```python
from build123d import *

# Parameters (mm, degrees)
SKETCH_2_W          = 60
SKETCH_2_H          = 95
EXTRUDE_1_DEPTH     = 45
SKETCH_3_W          = 56
SKETCH_3_H          = 91
CUT_EXTRUDE_1_DEPTH = 40
SKETCH_5_W          = 51
SKETCH_5_H          = 70
CUT_EXTRUDE_2_DEPTH = 5
SKETCH_6_R          = 1.5
CUT_EXTRUDE_3_DEPTH = 5
SKETCH_8_R          = 2.75
CUT_EXTRUDE_4_DEPTH = 2.5
SKETCH_10_W         = 36
SKETCH_10_H         = 3
CUT_EXTRUDE_5_DEPTH = 2
SKETCH_11_W         = 60
SKETCH_11_H         = 95
EXTRUDE_2_DEPTH     = 5
SKETCH_12_W         = 56
SKETCH_12_H         = 91
CUT_EXTRUDE_6_DEPTH = 5
SKETCH_13_W         = 9
SKETCH_13_H         = 11
CUT_EXTRUDE_7_DEPTH = 5
SKETCH_14_W         = 22
SKETCH_14_H         = 19
EXTRUDE_3_DEPTH     = 31
SKETCH_15_W         = 20
SKETCH_15_H         = 17
CUT_EXTRUDE_8_DEPTH = 30
SKETCH_16_W         = 16
SKETCH_16_H         = 14
CUT_EXTRUDE_9_DEPTH = 2


with BuildPart() as part:
    # 草圖2 → 填料-伸長1 (new body)
    with BuildSketch(Plane(origin=(0, 0, 0), x_dir=(1, 0, 0), z_dir=(0, 1, 0))):
        with Locations((30, 47.5)):
            Rectangle(SKETCH_2_W, SKETCH_2_H)
    extrude(amount=EXTRUDE_1_DEPTH)

    # 草圖3 → 除料-伸長1 (cut)
    with BuildSketch(Plane(origin=(0, 45, 0), x_dir=(1, 0, 0), z_dir=(0, 1, 0))):
        with Locations((30, 47.5)):
            Rectangle(SKETCH_3_W, SKETCH_3_H)
    extrude(amount=-CUT_EXTRUDE_1_DEPTH, mode=Mode.SUBTRACT)

    # 草圖5 → 除料-伸長2 (cut)
    with BuildSketch(Plane(origin=(0, 5, 0), x_dir=(1, 0, 0), z_dir=(0, 1, 0))):
        with Locations((30, 46.5)):
            Rectangle(SKETCH_5_W, SKETCH_5_H)
    extrude(amount=-CUT_EXTRUDE_2_DEPTH, mode=Mode.SUBTRACT)

    # 草圖6 → 除料-伸長3 (cut)
    with BuildSketch(Plane(origin=(0, 5, 0), x_dir=(1, 0, 0), z_dir=(0, 1, 0))):
        with Locations(Location((8, 8.5, 0), (0, 0, 270))):  # turned: the seam where the file's is
            Circle(SKETCH_6_R)
        with Locations(Location((52, 8.5, 0), (0, 0, 270))):  # turned: the seam where the file's is
            Circle(SKETCH_6_R)
        with Locations(Location((8, 84.5, 0), (0, 0, 270))):  # turned: the seam where the file's is
            Circle(SKETCH_6_R)
        with Locations(Location((52, 84.5, 0), (0, 0, 270))):  # turned: the seam where the file's is
            Circle(SKETCH_6_R)
    extrude(amount=-CUT_EXTRUDE_3_DEPTH, mode=Mode.SUBTRACT)

    # 草圖8 → 除料-伸長4 (cut)
    with BuildSketch(Plane(origin=(0, 0, 0), x_dir=(-1, 0, 0), z_dir=(0, -1, 0))):
        with Locations(Location((-8, 84.5, 0), (0, 0, 90))):  # turned: the seam where the file's is
            Circle(SKETCH_8_R)
        with Locations(Location((-8, 8.5, 0), (0, 0, 90))):  # turned: the seam where the file's is
            Circle(SKETCH_8_R)
        with Locations(Location((-52, 8.5, 0), (0, 0, 90))):  # turned: the seam where the file's is
            Circle(SKETCH_8_R)
        with Locations(Location((-52, 84.5, 0), (0, 0, 90))):  # turned: the seam where the file's is
            Circle(SKETCH_8_R)
    extrude(amount=-CUT_EXTRUDE_4_DEPTH, mode=Mode.SUBTRACT)

    # 草圖10 → 除料-伸長5 (cut)
    with BuildSketch(Plane(origin=(0, 5, 0), x_dir=(1, 0, 0), z_dir=(0, 1, 0))):
        with Locations((30, 89.5)):
            Rectangle(SKETCH_10_W, SKETCH_10_H)
    extrude(amount=-CUT_EXTRUDE_5_DEPTH, mode=Mode.SUBTRACT)

    # 草圖11 → 填料-伸長2 (add)
    with BuildSketch(Plane.XZ.offset(-45)):
        with Locations((30, -47.5)):
            Rectangle(SKETCH_11_W, SKETCH_11_H)
    extrude(amount=-EXTRUDE_2_DEPTH)

    # 草圖12 → 除料-伸長6 (cut)
    with BuildSketch(Plane(origin=(0, 50, 0), x_dir=(1, 0, 0), z_dir=(0, 1, 0))):
        with Locations((30, 47.5)):
            Rectangle(SKETCH_12_W, SKETCH_12_H)
    extrude(amount=-CUT_EXTRUDE_6_DEPTH, mode=Mode.SUBTRACT)

    # 草圖13 → 除料-伸長7 (cut)
    with BuildSketch(Plane.ZY):
        with Locations((-62.5, 27.2)):
            Rectangle(SKETCH_13_W, SKETCH_13_H)
    extrude(amount=-CUT_EXTRUDE_7_DEPTH, mode=Mode.SUBTRACT)

    # 草圖14 → 填料-伸長3 (add)
    with BuildSketch(Plane.XY):
        with Locations((30, 29.5)):
            Rectangle(SKETCH_14_W, SKETCH_14_H)
    extrude(amount=-EXTRUDE_3_DEPTH)

    # 草圖15 → 除料-伸長8 (cut)
    with BuildSketch(Plane.XY):
        with Locations((30, 29.5)):
            Rectangle(SKETCH_15_W, SKETCH_15_H)
    extrude(amount=-CUT_EXTRUDE_8_DEPTH, mode=Mode.SUBTRACT)

    # 草圖16 → 除料-伸長9 (cut)
    with BuildSketch(Plane(origin=(0, 39, 0), x_dir=(1, 0, 0), z_dir=(0, 1, 0))):
        with Locations((30, 22)):
            Rectangle(SKETCH_16_W, SKETCH_16_H)
    extrude(amount=-CUT_EXTRUDE_9_DEPTH, mode=Mode.SUBTRACT)


solid = part.part
```
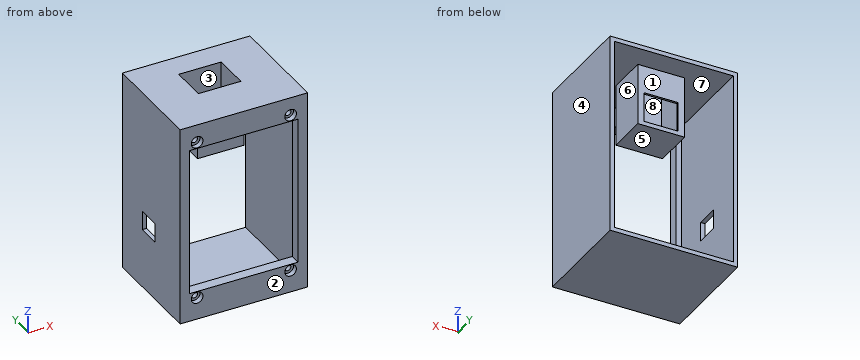
The model under review builds one solid part; all positions refer to its coordinate system, in mm. Face numbers are marked on the shaded views. A direction names the side the tool comes from. Give positions to 0.01 mm unless a question says otherwise; leave off trailing zeros. Write each loop counter-clockwise with the first axis right and the second up, starting at its lowest first coordinate (ties: lowest second). Pieces come first, ordered by that corner, then holes.
(1) Tool access review of the marked faces 5, 6, 7 and 8: name each direction out of +Z, -Z, +X, -X, +Y, -Y from which nothing blocks a thin tool from reaching the whole face with its end or side.
(2) The part is to be moulded in two halves that separate along Y. For the marked faces 1, 2, 3 and 4, say which applies: released by +Y, released by -Y, zero draft, split by the parting line, or undercut.
(3) Consider section C-C, the plane x = 8. Give the boundary of the cut face in (y, z).
(4) Consider section B-B, the plane z = -8.5. Give the number of separate pieces and of enclosed holes in the cut face, and give its area (4 significant figures).
(5) To check wall thickness, follow L1, parallel to X at y = 33, z = -14; L2, parallel to X at y = 4.05, z = -84.5; L3, parallel to Z at x = 24, y = 38.5. State the ranges of each line that lie inside material, in increasing order.
(6) Consider section D-D, the plane z = -19. Give the boundary of the cut face in (x, y).
(7) For P1, Ø4, axis at y = 12, z = -11, coming from the -X side; P2, Ø4.5, axis at x = 52, z = -8.5, coming from the +Y side; P3, Ø0.9, axis at x = 23.5, z = -89.5, coming from the +Y side; P4, Ø1.5, axis at x = 32, z = -21.5, coming from the +Y side, all flat-tipped, find the tip position at first contact; note any pin that passes through.
(8) Consider section A-A, the plane x = 16. Give the boundary of the cut face in (y, z), and give its area (3 significant figures).
Returned:
1. face 5: +Y, -Y
1. face 6: +Y
1. face 7: none
1. face 8: +Z
2. face 1: released by +Y
2. face 2: released by -Y
2. face 3: undercut
2. face 4: zero draft
3. outline: (0, -95) - (50, -95) - (50, -93) - (5, -93) - (5, -86) - (2.5, -86) - (2.5, -87.25) - (0, -87.25) - close; (0, -81.75) - (2.5, -81.75) - (2.5, -83) - (5, -83) - (5, -81.5) - (0, -81.5) - close; (0, -11.5) - (5, -11.5) - (5, -10) - (2.5, -10) - (2.5, -11.25) - (0, -11.25) - close; (0, -5.75) - (2.5, -5.75) - (2.5, -7) - (5, -7) - (5, -2) - (50, -2) - (50, 0) - (0, 0) - close
4. separate pieces: 4
4. enclosed holes: 1
4. area: 515.5 mm2
5. L1: x = 0 to 2, 19 to 20, 40 to 41, 58 to 60
5. L2: x = 0 to 6.5, 9.5 to 50.5, 53.5 to 60
5. L3: z = -95 to -93, -31 to -29, -15 to 0
6. outline: (0, 0) - (4.5, 0) - (4.5, 5) - (2, 5) - (2, 50) - (0, 50) - close; (19, 20) - (41, 20) - (41, 39) - (38, 39) - (38, 38) - (40, 38) - (40, 21) - (20, 21) - (20, 38) - (22, 38) - (22, 39) - (19, 39) - close; (55.5, 0) - (60, 0) - (60, 50) - (58, 50) - (58, 5) - (55.5, 5) - close
7. P1: stops at x = 0
7. P2: stops at y = 5
7. P3: stops at y = 3
7. P4: stops at y = 21
8. outline: (0, -95) - (50, -95) - (50, -93) - (5, -93) - (5, -91) - (3, -91) - (3, -88) - (5, -88) - (5, -81.5) - (0, -81.5) - close; (0, -11.5) - (5, -11.5) - (5, -2) - (50, -2) - (50, 0) - (0, 0) - close
8. area: 299 mm2
